Source: CAD feature listing. Evaluate the final solid. Frame: model axes, mm. Face numbers are marked on the shaded views. A direction names the side the tool comes from. Round coordinates to 2 decimals unless told otherwise and drop trailing zeros. Loops run counter-clockwise (first coordinate to the right, second up) from the corner with the lowest first, then second, coordinate; pieces in that order, holes last. Notation, with made-up numbers: (45.5, -10.75) - (63.5, -10.75) arc R20 ccw to (63.5, 10.25) - close; hole circle Ø8 at (5, 37.5). An arc over 180 degrees is marked (long way). Write item = value, one per line. Start each with the question number.
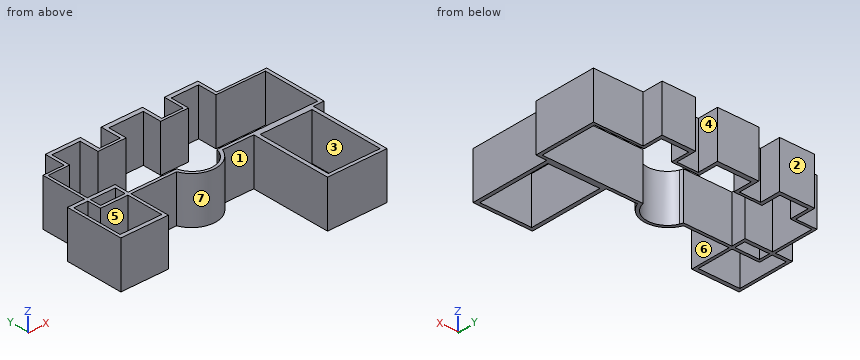
from build123d import *

# Parameters (mm, degrees)
F0_W     = 1.4990121126
F0_H     = 1.9831014797
F0_W_2   = 1.6156211495
F0_H_2   = 1.6615597997
F0_W_3   = 28.149546124
F0_H_3   = 40.3955862857
F1_DEPTH = 25.4


with BuildPart() as f1:
    # F0 (on Top) → F1 (new body)
    with BuildSketch(Plane.XY):
        Polygon((-11.7408363149, 45.5303452909), (-11.7408363149, 34.1073982418), (-9.8901251331, 34.1073982418), (-9.8901251331, 43.0053770542), (8.778876625, 43.0053770542), (8.778876625, 34.1073982418), (10.634101578, 34.1073982418), (10.634101578, 45.5303452909), align=None)
        Polygon((-42.2627404332, 45.3080944717), (-42.2627404332, 34.1073982418), (-40.5606254935, 34.1073982418), (-40.5606254935, 43.2276241481), (-25.2253748477, 43.2276241481), (-25.2253748477, 34.1073982418), (-23.2215542346, 34.1073982418), (-23.2215542346, 45.3080944717), align=None)
        Polygon((-23.2215542346, 34.1073982418), (-25.2253748477, 34.1073982418), (-25.2253748477, 32.7079482377), (-9.8901251331, 32.7079482377), (-9.8901251331, 34.1073982418), (-11.7408363149, 34.1073982418), align=None)
        Polygon((-42.2627404332, 34.1073982418), (-53.743455559, 34.1073982418), (-53.743455559, 9.4658602029), (-52.2444434464, 9.4658602029), (-52.2444434464, 32.7079482377), (-40.5606254935, 32.7079482377), (-40.5606254935, 34.1073982418), align=None)
        Polygon((-53.743455559, 7.4827587232), (-53.743455559, 9.4658602029), (-62.9840344191, 9.4658602029), (-62.9840344191, -22.1761129797), (-37.2224263847, -22.1761129797), (-37.2224263847, 0), (-38.8380475342, 0), (-38.8380475342, -20.0356338173), (-61.4172406495, -20.0356338173), (-61.4172406495, 7.4827587232), align=None)
        Polygon((-52.2444434464, 7.4827587232), (-53.743455559, 7.4827587232), (-53.743455559, 0), (-38.8380475342, 0), (-38.8380475342, 1.6615597997), (-52.2444434464, 1.6615597997), align=None)
        Polygon((-37.2224263847, 9.4658602029), (-52.2444434464, 9.4658602029), (-52.2444434464, 7.4827587232), (-38.8380475342, 7.4827587232), (-38.8380475342, 1.6615597997), (-37.2224263847, 1.6615597997), align=None)
        with Locations((-52.9939495027, 8.4743094631)):
            Rectangle(F0_W, F0_H)
        with Locations((-38.0302369595, 0.8307798998)):
            Rectangle(F0_W_2, F0_H_2)
        with BuildLine():
            Line((-10.9551865608, 1.6615597997), (-37.2224263847, 1.6615597997))
            Line((-37.2224263847, 1.6615597997), (-37.2224263847, 0))
            Line((-37.2224263847, 0), (-12.4503001571, 0))
            Line((-12.4503001571, 0), (-10.4229850138, 0))
            ThreePointArc((-10.4229850138, 0), (-10.7213890086, 0.8204331014), (-10.9551865608, 1.6615597997))
        make_face()
        with BuildLine():
            Line((31.4435763285, 1.6615597997), (10.9108546749, 1.6615597997))
            ThreePointArc((10.9108546749, 1.6615597997), (10.6770571227, 0.8204331014), (10.378653128, 0))
            Line((10.378653128, 0), (12.4059682712, 0))
            Line((12.4059682712, 0), (29.3507482857, 0))
            Line((29.3507482857, 0), (31.4435763285, 0))
            Line((31.4435763285, 0), (31.4435763285, 1.6615597997))
        make_face()
        with BuildLine():
            Line((-10.4229850138, 0), (-12.4503001571, 0))
            ThreePointArc((-12.4503001571, 0), (-0.0221659429, -8.5303409081), (12.4059682712, 0))
            Line((12.4059682712, 0), (10.378653128, 0))
            ThreePointArc((10.378653128, 0), (-0.0221659429, -6.9872415007), (-10.4229850138, 0))
        make_face()
        Polygon((31.4435763285, 0), (29.3507482857, 0), (29.3507482857, -43.7374562025), (61.623737216, -43.7374562025), (61.623737216, 0), align=None)
        with Locations((45.5183493905, -21.7114321422)):
            Rectangle(F0_W_3, F0_H_3, mode=Mode.SUBTRACT)
        Polygon((65.5907168984, 1.6615597997), (31.4435763285, 1.6615597997), (31.4435763285, 0), (61.623737216, 0), (67.5041079521, 0), (67.5041079521, 34.1073982418), (40.482412558, 34.1073982418), (38.7573502958, 34.1073982418), (38.7573502958, 32.7079482377), (65.5907168984, 32.7079482377), align=None)
        Polygon((22.2812830471, 34.1073982418), (23.8918736577, 34.1073982418), (23.8918736577, 43.0053770542), (38.7573502958, 43.0053770542), (38.7573502958, 34.1073982418), (40.482412558, 34.1073982418), (40.482412558, 45.3080944717), (22.2812830471, 45.3080944717), align=None)
        Polygon((8.778876625, 34.1073982418), (8.778876625, 32.7079482377), (23.8918736577, 32.7079482377), (23.8918736577, 34.1073982418), (22.2812830471, 34.1073982418), (10.634101578, 34.1073982418), align=None)
    extrude(amount=F1_DEPTH)


solid = f1.part
(1) Access query for the marked faces 1, 2, 3 and 4. Directions: +Z, -Z, +X, -X, +Y, -Y. A direction counts if a zero-diameter tool reaches every point of the face in a straight line with its end or side. Return the directions, or none.
(2) Cut plane B-B (x = 57.5). Output: boundary loops of the cut face in (y, z).
(3) Cut plane D-D (x = -18.5). Output: boundary loops of the cut face in (y, z).
(4) Cut plane C-C (y = 15). Output: boundary loops of the cut face in (x, z), and give its area (3 significant figures).
(5) Mould query, pull axis Y, two halves, no side actions, for the marked faces 5, 6 and 7. Classes: +Y half, -Y half, draft (parallel to the pull), parting line (faces both ways), or undercut.
(6) Material intervals for line 1 along Y through (x, z) = (-48, 23.5); line 2 along Y through (x, z) = (45, 3.5); line 3 along X through (y, z) = (-10, 12.75), sorted ascending. Write a range as from..to.
(7) Cut plane A-A (y = -10). Output: boundary loops of the cut face in (x, z).
(8) Pin query (flat end, axial travel): P1, Ø12.5, axis at y = -18, z = 7.5, coming from the +X side; P2, Ø10, axis at x = -47.5, z = 2.5, coming from the +Y side; P3, Ø4, axis at x = -45, z = 11.5, coming from the -Y side; P4, Ø8, axis at x = -48.5, y = -5, coming from the -Z side. Return the tip coordinate at first contact, or that it passes through.
Solution:
q1.face_1 = +Z, -Z, -Y
q1.face_2 = +Z, -Z, -X, +Y
q1.face_3 = +Z, -Z
q1.face_4 = +Z, -Z, +Y
q2.outline = (-43.74, 0) - (-41.91, 0) - (-41.91, 25.4) - (-43.74, 25.4) - close; (-1.51, 0) - (1.66, 0) - (1.66, 25.4) - (-1.51, 25.4) - close; (32.71, 0) - (34.11, 0) - (34.11, 25.4) - (32.71, 25.4) - close
q3.outline = (0, 0) - (1.66, 0) - (1.66, 25.4) - (0, 25.4) - close; (32.71, 0) - (34.11, 0) - (34.11, 25.4) - (32.71, 25.4) - close
q4.outline = (-53.74, 0) - (-52.24, 0) - (-52.24, 25.4) - (-53.74, 25.4) - close; (65.59, 0) - (67.5, 0) - (67.5, 25.4) - (65.59, 25.4) - close
q4.area = 86.7 mm^2
q5.face_5 = undercut
q5.face_6 = draft
q5.face_7 = -Y half
q6.line_1 = -22.18..-20.04, 0..1.66, 7.48..9.47, 32.71..34.11
q6.line_2 = -43.74..-41.91, -1.51..1.66, 32.71..34.11
q6.line_3 = -62.98..-61.42, -38.84..-37.22, 29.35..31.44, 59.59..61.62
q7.outline = (-62.98, 0) - (-61.42, 0) - (-61.42, 25.4) - (-62.98, 25.4) - close; (-38.84, 0) - (-37.22, 0) - (-37.22, 25.4) - (-38.84, 25.4) - close; (29.35, 0) - (31.44, 0) - (31.44, 25.4) - (29.35, 25.4) - close; (59.59, 0) - (61.62, 0) - (61.62, 25.4) - (59.59, 25.4) - close
q8.P1 = 61.62
q8.P2 = 34.11
q8.P3 = -22.18
q8.P4 = through
